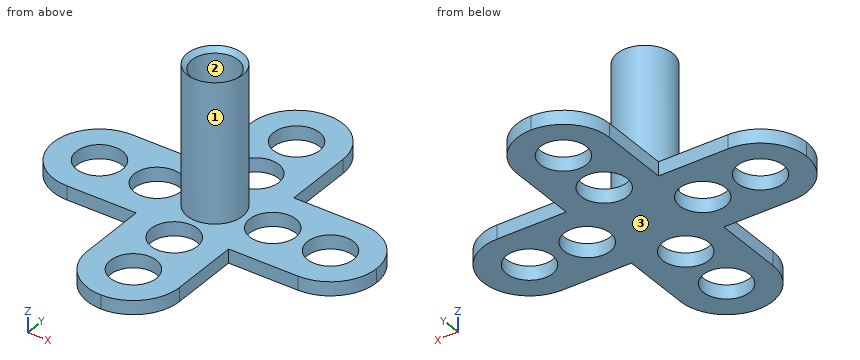
```python
from build123d import *

# Parameters (mm, degrees)
F1_DEPTH = 3
F3_D     = 10
F4_R     = 6
F4_R_2   = 5
F5_DEPTH = 30
F6_SIZE  = 0.99999


# Not quite as in the source:
# - a fillet or chamfer is up to 0.001 mm smaller than in the source, because OpenCascade refuses the exact size


with BuildPart() as f1:
    # F0 (on Top) → F1 (new body)
    with BuildSketch(Plane.XY):
        with BuildLine():
            Line((10, 10), (10, 25))
            ThreePointArc((10, 25), (7.0710678119, 32.0710678119), (0, 35))
            ThreePointArc((0, 35), (-7.0710678119, 32.0710678119), (-10, 25))
            Line((-10, 25), (-10, 10))
            Line((-10, 10), (-25, 10))
            ThreePointArc((-25, 10), (-32.0710678119, 7.0710678119), (-35, 0))
            ThreePointArc((-35, 0), (-32.0710678119, -7.0710678119), (-25, -10))
            Line((-25, -10), (-10, -10))
            Line((-10, -10), (-10, -25))
            ThreePointArc((-10, -25), (-7.0710678119, -32.0710678119), (0, -35))
            ThreePointArc((0, -35), (7.0710678119, -32.0710678119), (10, -25))
            Line((10, -25), (10, -10))
            Line((10, -10), (25, -10))
            ThreePointArc((25, -10), (32.0710678119, -7.0710678119), (35, 0))
            ThreePointArc((35, 0), (32.0710678119, 7.0710678119), (25, 10))
            Line((25, 10), (10, 10))
        make_face()
    extrude(amount=F1_DEPTH)

    # F3 (through all)
    with Locations(Plane.XY.offset(3)):
        with Locations((-25, 0), (-12.5, 0), (0, 25), (0, 12.5), (12.5, 0), (25, 0), (0, -12.5), (0, -25)):
            Hole(F3_D / 2)

    # F4 (on face) → F5 (join)
    with BuildSketch(Plane.XY.offset(3)):
        Circle(F4_R)
        Circle(F4_R_2, mode=Mode.SUBTRACT)
    extrude(amount=F5_DEPTH)

    # F6 (size 1 in the source; OpenCascade refuses exactly that, so slightly less here)
    f6_edges = [f1.edges().sort_by_distance(p)[0] for p in [
        (-5, 0, 33),
    ]]
    chamfer(f6_edges, length=F6_SIZE)


solid = f1.part
```
Build history of the part. All positions in model axes, mm. Face numbers are marked on the shaded views. Round coordinates to 2 decimals unless told otherwise and drop trailing zeros. Write each loop counter-clockwise with the first axis right and the second up, starting at its lowest first coordinate (ties: lowest second). Pieces come first, ordered by that corner, then holes. Notation, with made-up numbers: (-17, 0) -> (41, 0) arc R26 cw to (41, 26) -> close; hole circle Ø3 at (-10, 31). An arc over 180 degrees is marked (long way). Put each result on its own line as item: value.
Item 1: Flat gauge pins, fed straight in: P1, Ø0.9, axis at y = -18.5, z = 1, coming from the +X side; P2, Ø6, axis at x = -11.5, y = 17.5, coming from the +Z side; P3, Ø11.5, axis at x = 0, y = -25, coming from the -Z side; P4, Ø1.5, axis at y = 18.5, z = 1, coming from the -X side. Where does each tip first touch, or does it go through?
Here are the results:
P1: stops at x = 10
P2: stops at z = 3
P3: stops at z = 0
P4: stops at x = -10
Item 2: Slice it at C-C, the plane z = 11.5. Give the cut face in (x, y), plus the area to 3 significant figures.
Here are the results:
outline: circle Ø12 at (0, 0); hole circle Ø10 at (0, 0)
area: 34.6 mm^2
Item 3: Wall check: probe 1 along Y at (x, z) = (-25, 1.25); probe 2 along X at (y, z) = (4, 22); probe 3 along Z at (x, y) = (7, 27). Give the ranges that are in metal, low to high. Write a range as from..to.
Here are the results:
probe 1: y = -10..-5, 5..10
probe 2: x = -4.47..-3, 3..4.47
probe 3: z = 0..3
Item 4: Slice it at A-A, the plane y = 12.5. Give the cut face in (x, z), plus the area to 3 significant figures.
Here are the results:
outline: (-10, 0) -> (-5, 0) -> (-5, 3) -> (-10, 3) -> close; (5, 0) -> (10, 0) -> (10, 3) -> (5, 3) -> close
area: 30.0 mm^2
Item 5: Two-plate mould, pull along X, no slides. Class the marked faces 1, 2 and 3: pulls with the +X half, pulls with the -X half, needs draft (parallel to the pull), parting line crosses it, or undercut.
Here are the results:
face 1: parting line crosses it
face 2: undercut
face 3: needs draft
